Work out the finished part from the listing and answer in its coordinate system (mm). Give positions to 0.01 mm unless a question says otherwise; leave off trailing zeros. Loops run counter-clockwise (first coordinate to the right, second up) from the corner with the lowest first, then second, coordinate; pieces in that order, holes last. Notation, with made-up numbers: (76.5, 75) -> (92.5, 75) arc R10 cw to (92.5, 80) -> close; hole circle Ø7 at (23, -32). An arc over 180 degrees is marked (long way). Answer as CSV lines item,"result". Start each with the question number.
1. Find section A-A, the plane y = -1.25. Give the vertices of the cut face in (x, z).
2. Find section C-C, the plane x = -2.75. Give the vertices of the cut face in (y, z), and give its area (3 significant figures).
3. Determine the mould class of faces 1 (the face through (0, -2, 0)), 2 (the face through (-0.1, -11.53, 2.46)), 3 (the face through (1.61, -0.34, 2.46)) for opening direction Y: +Y half, -Y half, draft (parallel to the pull), parting line (faces both ways), or undercut.
4. Find the intervals of material crossed by line 1 along Y through (x, z) = (-0.25, 0.8); line 2 along Y through (x, z) = (-2.75, 3.9); line 3 along X through (y, z) = (-3.25, 3.5), in increasing order.
5. Find section B-B, the plane x = 6.5. Give the vertices of the cut face in (y, z).
6. Find section D-D, the plane y = -10. Give the vertices of the cut face in (x, z), and give its area (3 significant figures).
7. Flat-ended cylindrical pins translate along their axes: pin 1 Ø2 at (x, z) = (6, 4.5) entering from -Y; pin 2 Ø3 at (y, z) = (-3, 1.5) entering from -X; pin 3 Ø1 at (y, z) = (-5.5, 1.5) entering from -X. Find the tip coordinate at first contact, or state that the pin passes through.
from build123d import *

# Parameters (mm, degrees)
F1_DEPTH = 5
F2_R     = 2


with BuildPart() as f1:
    # F0 (on Top) → F1 (new body)
    with BuildSketch(Plane.XY):
        with BuildLine():
            ThreePointArc((-9.125, -12.559485), (0, -11.531155), (9.125, -12.559485))
            ThreePointArc((9.125, -12.559485), (10.96678, -3.563323), (14.76456, 4.797296))
            ThreePointArc((14.76456, 4.797296), (6.777843, 9.3289), (0, 15.524377))
            ThreePointArc((0, 15.524377), (-6.777843, 9.3289), (-14.76456, 4.797296))
            ThreePointArc((-14.76456, 4.797296), (-10.96678, -3.563323), (-9.125, -12.559485))
        make_face()
        with BuildLine():
            ThreePointArc((-6.594019, 5.336478), (8.615573, -0.177029), (-6.594019, -5.690536))
            ThreePointArc((-6.594019, -5.690536), (1.613356, -0.177029), (-6.594019, 5.336478))
        make_face(mode=Mode.SUBTRACT)
    extrude(amount=F1_DEPTH)

    # F2
    f2_edges = [f1.edges().sort_by_distance(p)[0] for p in [
        (-14.76456, 4.797296, 2.5),
        (0, 15.524377, 2.5),
        (14.76456, 4.797296, 2.5),
        (9.125, -12.559485, 2.5),
        (-9.125, -12.559485, 2.5),
    ]]
    fillet(f2_edges, radius=F2_R)


solid = f1.part
Resolved:
1,outline,"(-11.8, 0) -> (1.52, 0) -> (1.52, 5) -> (-11.8, 5) -> close; (8.55, 0) -> (11.8, 0) -> (11.8, 5) -> (8.55, 5) -> close"
2,outline,"(-11.62, 0) -> (-8.33, 0) -> (-8.33, 5) -> (-11.62, 5) -> close; (-5.92, 0) -> (5.56, 0) -> (5.56, 5) -> (-5.92, 5) -> close; (7.97, 0) -> (12.67, 0) -> (12.67, 5) -> (7.97, 5) -> close"
2,area,"97.4 mm^2"
3,face 1,"draft"
3,face 2,"-Y half"
3,face 3,"undercut"
4,line 1,"y = -11.53 to -8.78, -4.5 to 4.15, 8.42 to 14.56"
4,line 2,"y = -11.62 to -8.33, -5.92 to 5.56, 7.97 to 12.67"
4,line 3,"x = -11.07 to 0.76, 8.05 to 11.07"
5,outline,"(-12.05, 0) -> (-5.83, 0) -> (-5.83, 5) -> (-12.05, 5) -> close; (5.47, 0) -> (9.53, 0) -> (9.53, 5) -> (5.47, 5) -> close"
6,outline,"(-9.44, 0) -> (9.44, 0) -> (9.44, 5) -> (-9.44, 5) -> close"
6,area,"94.4 mm^2"
7,pin 1,"stops at y = -12.13"
7,pin 2,"stops at x = -11.7"
7,pin 3,"stops at x = -10.53"
